Read the model definition and answer for the solid it produces. Units are mm, in the model's axes. A direction names the side the tool comes from. Coordinates: 2 decimals unless noted, no trailing zeros. Loops run counter-clockwise (first coordinate to the right, second up) from the corner with the lowest first, then second, coordinate; pieces in that order, holes last. Notation, with made-up numbers: (1.25, 79.5) - (33.25, 79.5) arc R29 ccw to (33.25, 100.5) - close; hole circle Ø6 at (22.25, 51). An arc over 180 degrees is marked (long way). One line per item, written item: value. Start each with the question number.
Autodesk Inventor part; units mm, degrees
ref_plane "YZ Plane" through (0, 0, 0) normal (1, 0, 0) x (0, 1, 0)
ref_plane "XZ Plane" through (0, 0, 0) normal (0, 1, 0) x (-1, 0, 0)
ref_plane "XY Plane" through (0, 0, 0) normal (0, 0, 1) x (1, 0, 0)
sketch "草图1" plane through (0, 0, 0) normal (1, 0, 0) x (0, 1, 0)
  line L0 (19.5, -23) -> (30, -23)
  line L1 (30, -23) -> (30, -68)
  line L2 (30, -68) -> (19.5, -68)
  line L3 (19.5, -68) -> (19.5, -78)
  line L4 (19.5, -78) -> (25, -78)
  line L5 (25, -78) -> (25, -206)
  line L6 (25, -206) -> (0, -206)
  line L7 (0, -206) -> (0, 0)
  line L8 (17.5, -16) -> (17.5, -9)
  line L9 (17.5, -9) -> (19.5, -9)
  line L10 (17.5, -16) -> (19.5, -16)
  line L11 (19.5, -16) -> (19.5, -23)
  line L12 (19.5, -23) -> (19.5, -6)
  line L13 (0, 0) -> (13.5, 0)
  arc A0 (19.5, -6) -> (13.5, 0) centre (8.1859, -11.3141) ccw
  dimension "d2" = 10.5
  dimension "d3" = 45
  dimension "d4" = 10.5
  dimension "d5" = 10
  dimension "d6" = 5.5
  dimension "d7" = 128
  dimension "d10" = 7
  dimension "d11" = 17
  dimension "d14" = 13.5
  dimension "d15" = 25
revolve "旋转1" add sketch "草图1" angle 360 about axis through (0, 0, -206) along (0, 0, 1) contours L0 L1 L2 L3 L4 L5 L6 L7 L13 A0 L12 L9 L8 L10 L11
sketch "草图2" plane through (0, 0, 0) normal (0, 1, 0) x (-1, 0, 0)
  line L0 (-19.5, -68) -> (19.5, -68)
  line L1 (0, -68) -> (0, -45.5)
  circle A0 centre (0, -45.5) radius 11
  point P0 (0, 0)
  dimension "d17" = 22.5
  dimension "d18" = 22
extrude "拉伸1" cut sketch "草图2" along normal blind 100 and the other way blind 100
thread "螺纹1"
sketch "草图3" plane through (0, 0, 0) normal (1, 0, 0) x (0, 1, 0)
  line L0 (-19.5, -68) -> (19.5, -68)
  line L1 (0, -68) -> (0, -45.5)
  circle A0 centre (0, -45.5) radius 11
  line L2 (-30, -34.5) -> (30, -34.5)
  point P0 (0, 0)
  dimension "d25" = 22.5
  dimension "d26" = 22
extrude "拉伸2" cut sketch "草图3" along normal blind 100 and the other way blind 50
properties part number "螺杆"
1) For faces 1 (the cylindrical face through (-18.124, -1.432, -34.594)), 2 (the flat face through (20, 0, -68)), 3 (the cylindrical face through (19.334, -2.539, -19.549)), 4 (the cylindrical face through (7.509, 23.846, -142.896)), determine the directions among +Z, -Z, +X, -X, +Y, -Y from which every point of the face is accessible in a straight line to the end or side of a thin tool.
2) Determine the mould class of faces 5 (the cylindrical face through (1.432, -18.124, -34.594)), 6 (the cylindrical face through (10.648, -13.887, -12.451)), 7 (the flat face through (20, 0, -23)) for opening direction X: released by +X, released by -X, zero draft, split by the parting line, or undercut.
3) Section A-A, the plane z = -45.5 is taken. Determine the outline of the cut face in (x, y).
4) Flat-ended cylindrical pins translate along their axes: P1, Ø8, axis at y = -23.5, z = -182.5, coming from the +X side; P2, Ø6, axis at y = -20, z = -32.5, coming from the +X side; P3, Ø8, axis at y = -16.5, z = -130.5, coming from the -X side. Find the tip coordinate at first contact, or state that the pin passes through.
5) Section B-B, the plane z = -177.5 is taken. Determine the outline of the cut face in (x, y), and give its area (3 significant figures).
6) Straight lines are drawn through the part: L1, parallel to Z at x = 0, y = -20; L2, parallel to Z at x = -17.5, y = 10; L3, parallel to Z at x = -18, y = -12.5. For each, find the intervals that lie inside material, in ascending order.
Answer below:
1. face 1: +X, -X
1. face 2: none
1. face 3: +Z
1. face 4: -Z
2. face 5: undercut
2. face 6: split by the parting line
2. face 7: zero draft
3. outline: (-27.91, -11) arc R30 ccw to (-11, -27.91) - (-11, -11) - close; (-27.91, 11) - (-11, 11) - (-11, 27.91) arc R30 ccw to start; (11, -27.91) arc R30 ccw to (27.91, -11) - (11, -11) - close; (11, 11) - (27.91, 11) arc R30 ccw to (11, 27.91) - close
4. P1: x = 15.64
4. P2: x = 24.72
4. P3: x = -21.65
5. outline: circle Ø50 at (0, 0)
5. area: 1,960 mm2
6. L1: -206 to -78, -68 to -56.5, -34.5 to -23
6. L2: -206 to -78, -68 to -50.08, -40.92 to -23
6. L3: -206 to -78, -68 to -23
